Can you work these out from the drawing? Everything is in mm from the part's minimum corner. Round coordinates to 2 decimals unless told otherwise and drop trailing zeros. Order: outer loops, then holes, each group sorted by start corner. A loop starts at its lowest first (then second) coordinate and runs counter-clockwise, first axis right, second up. Notation, with made-up numbers: (3.25, 75.5) - (59.25, 75.5) arc R13 cw to (59.25, 87.5) - close; hole circle Ø6 at (2.25, -30.5). An arc over 180 degrees is marked (long way). Answer as a JSON object with one key per item and string values.
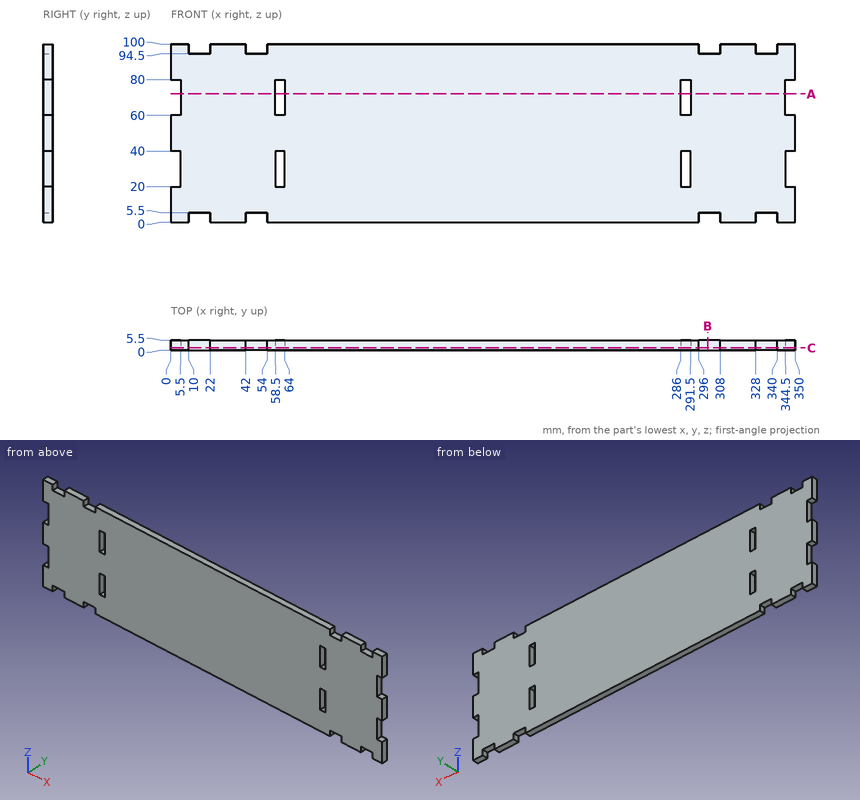
1. For P1, Ø3, axis at x = 301, y = 2.5, coming from the -Z side; P2, Ø1, axis at y = 2, z = 68.5, coming from the +X side; P3, Ø3, axis at y = 2.5, z = 32.5, coming from the -X side, each with a flat end and sliding along its axis, tell me the tip position at first contact or that it passes through.
Responses:
{"P1": "z = 5.5", "P2": "x = 344.5", "P3": "x = 5.5"}
2. Imagine slicing it at B-B (x = 301). List the corners of the cut face in (y, z) for me.
Responses:
{"outline": "(0, 5.5) - (5.5, 5.5) - (5.5, 94.5) - (0, 94.5) - close"}
3. Imagine slicing it at A-A (z = 72). List the corners of the cut face in (x, y) for me.
Responses:
{"outline": "(5.5, 0) - (58.5, 0) - (58.5, 5.5) - (5.5, 5.5) - close; (64, 0) - (286, 0) - (286, 5.5) - (64, 5.5) - close; (291.5, 0) - (344.5, 0) - (344.5, 5.5) - (291.5, 5.5) - close"}
4. If I drill on L1, parallel to X at y = 2.1, z = 39; L2, parallel to Z at x = 53, y = 3, over which ranges is the centre line in solid material (lowest first)? Write a range as [from, to].
Responses:
{"L1": "[5.5, 58.5], [64, 286], [291.5, 344.5]", "L2": "[5.5, 94.5]"}
5. Imagine slicing it at C-C (y = 1.25). Give the number of separate pieces and of enclosed holes in the cut face, plus the area to 3 significant figures.
Responses:
{"separate pieces": "1", "enclosed holes": "4", "area": "33,600 mm2"}
